from build123d import *

# Parameters (mm, degrees)
F0_W          = 15
F0_H          = 20
F1_DEPTH      = 26
F2_R          = 3
F3_DEPTH      = 10.001
F3_DEPTH_BACK = 10.001
F4_R          = 3
F5_DEPTH      = 7.501
F5_DEPTH_BACK = 7.501
F6_W          = 4.5
F6_H          = 14
F7_DEPTH      = 10.001
F7_DEPTH_BACK = 10.001
F8_W          = 15
F8_H          = 30
F9_DEPTH      = 3
F10_R         = 2


# Not quite as in the source:
# - two fillets or chamfers of one size are made in one step
# - a feature names something its author has since deleted; it is built from what else it names


with BuildPart() as f1:
    # F0 (on Top) → F1 (new body)
    with BuildSketch(Plane.XY):
        Rectangle(F0_W, F0_H)
    extrude(amount=F1_DEPTH)

    # F2 (on Front) → F3 (cut, two sides)
    with BuildSketch(Plane.XZ) as f3_sk:
        with Locations((0, 7)):
            Circle(F2_R)
    extrude(amount=-F3_DEPTH, mode=Mode.SUBTRACT)
    extrude(f3_sk.sketch, amount=F3_DEPTH_BACK, mode=Mode.SUBTRACT)

    # F4 (on Right) → F5 (cut, two sides)
    with BuildSketch(Plane.YZ) as f5_sk:
        with Locations((0, 21)):
            Circle(F4_R)
    extrude(amount=-F5_DEPTH, mode=Mode.SUBTRACT)
    extrude(f5_sk.sketch, amount=F5_DEPTH_BACK, mode=Mode.SUBTRACT)

    # F6 (on Front) → F7 (cut, two sides)
    with BuildSketch(Plane.XZ) as f7_sk:
        with Locations((0, 19)):
            Rectangle(F6_W, F6_H)
    extrude(amount=-F7_DEPTH, mode=Mode.SUBTRACT)
    extrude(f7_sk.sketch, amount=F7_DEPTH_BACK, mode=Mode.SUBTRACT)

    # F8 (on face) → F9 (join)
    with BuildSketch(Plane(origin=(0, 0, 0), x_dir=(1, 0, 0), z_dir=(0, 0, -1))):
        with Locations((0, -5)):
            Rectangle(F8_W, F8_H)
    extrude(amount=F9_DEPTH)

    # F10
    f10_edges = [f1.edges().sort_by_distance(p)[0] for p in [
        (7.5, -10, 11.5),
        (-7.5, -10, 11.5),
        (-7.5, 10, 13),
        (7.5, 10, 13),
        (2.25, 0, 12),
        (-2.25, 0, 12),
    ]]
    fillet(f10_edges, radius=F10_R)


solid = f1.part
Here's how the part is built. I have some questions about the finished solid (model axes, mm). A direction names the side the tool comes from. Give positions to 0.01 mm unless a question says otherwise; leave off trailing zeros. Order: outer loops, then holes, each group sorted by start corner. A loop starts at its lowest first (then second) coordinate and runs counter-clockwise, first axis right, second up. Notation, with made-up numbers: M 40,7 L 80,7 A19 cw 80,23 Z; hole C 41.5,42.5 d8. An arc over 180 degrees is marked long. Answer as a JSON object with one key per item and string values. Group by question number.
1) Suppose I cut it at A-A, the plane z = 21. Write out the boundary of the cut face in (x, y).
2) Please list where these lines run through material, in increasing order: L1, parallel to Z at x = 6.05, y = 0; L2, parallel to Z at x = 0, y = -7; L3, parallel to X at y = -4, z = 7. Write a range as [from, to].
3) Suppose I cut it at B-B, the plane x = -4.75. Write out the boundary of the cut face in (y, z), plus the area to 3 significant figures.
4) On a 3-axis mill with a long thin cutter (end or side, diameter ignored), from which of +Z, -Z, +X, -X, +Y, -Y can I reach the whole of each face in a straight line? I mean faces 4 (the cylindrical face through (-1.68, -0.14, 12.6)), 5 (the cylindrical face through (-6.93, 9.4, 13.18)), 6 (the flat face through (7.5, 0, 12)). Say none if no direction works.
5) I'm going to push flat-ended pins straight in: pin 1 Ø3.5 at (x, z) = (0, 7) entering from +Y; pin 2 Ø13 at (y, z) = (-1, 19.5) entering from +X; pin 3 Ø6 at (x, y) = (-2, 15.5) entering from +Z; pin 4 Ø3.5 at (x, z) = (1.5, 7.5) entering from +Y. Where does each tip first touch, or does it pass through?
6) Suppose I cut it at C-C, the plane x = -1. Write out the boundary of the cut face in (y, z).
7) We'd pull the mould along X, two halves only. Please class faces 1 (the cylindrical face through (6.93, 9.4, 13.18)), 2 (the cylindrical face through (1.65, -0.14, 12.57)), 3 (the flat face through (-7.5, 0, 12)): pulls with the +X half, pulls with the -X half, needs draft (parallel to the pull), parting line crosses it, or undercut.
8) Suppose I cut it at D-D, the plane z = 1.5. Write out the boundary of the cut face in (x, y), plus the area to 3 significant figures.
Results found:
{
 "1": {"outline": "M -7.5,-8 A2 ccw -5.5,-10 L -2.25,-10 L -2.25,-3 L -7.5,-3 Z; M -7.5,3 L -2.25,3 L -2.25,10 L -5.5,10 A2 ccw -7.5,8 Z; M 2.25,-10 L 5.5,-10 A2 ccw 7.5,-8 L 7.5,-3 L 2.25,-3 Z; M 2.25,3 L 7.5,3 L 7.5,8 A2 ccw 5.5,10 L 2.25,10 Z"},
 "2": {"L1": "[-3, 18], [24, 26]", "L2": "[-3, 4], [10, 12]", "L3": "[-7.5, -3], [3, 7.5]"},
 "3": {"outline": "M -10,-3 L 20,-3 L 20,0 L 10,0 L 10,26 L -10,26 Z; hole C 0,21 d6", "area": "582 mm²"},
 "4": {"face 4": "+Z, +Y, -Y", "face 5": "+Z, -X, +Y", "face 6": "+Z, -Z, +X, +Y, -Y"},
 "5": {"pin 1": "through", "pin 2": "x = 7.5", "pin 3": "z = 0", "pin 4": "y = 10"},
 "6": {"outline": "M -10,-3 L 20,-3 L 20,0 L 10,0 L 10,4.17 L -10,4.17 Z; M -10,9.83 L 10,9.83 L 10,12.15 L -10,12.15 Z"},
 "7": {"face 1": "pulls with the +X half", "face 2": "undercut", "face 3": "pulls with the -X half"},
 "8": {"outline": "M -7.5,-8 A2 ccw -5.5,-10 L 5.5,-10 A2 ccw 7.5,-8 L 7.5,8 A2 ccw 5.5,10 L -5.5,10 A2 ccw -7.5,8 Z", "area": "297 mm²"}
}
